Verification items for the finished model (mm, model axes). A direction names the side the tool comes from. Coordinates: 2 decimals unless noted, no trailing zeros. Write each loop counter-clockwise with the first axis right and the second up, starting at its lowest first coordinate (ties: lowest second). Pieces come first, ordered by that corner, then holes. Notation, with made-up numbers: (72.25, -7) - (97.25, -7) arc R25 cw to (97.25, 31) - close; hole circle Ø8 at (24.5, 18). An arc over 180 degrees is marked (long way). Answer as CSV lines item,"result". Start each with the question number.
```python
from build123d import *

# Parameters (mm, degrees)
SKETCH1_W           = 100
SKETCH1_H           = 100
SKETCH1_R           = 16.5
BOSS_EXTRUDE1_DEPTH = 10
SKETCH3_W           = 80
SKETCH3_H           = 80
SKETCH3_W_2         = 72
SKETCH3_H_2         = 72
BOSS_EXTRUDE2_DEPTH = 10


with BuildPart() as part:
    # Sketch1 → Boss-Extrude1 (new body)
    with BuildSketch(Plane(origin=(0, 0, 0), x_dir=(1, 0, 0), z_dir=(0, 1, 0))):
        Rectangle(SKETCH1_W, SKETCH1_H)
        with Locations(Location((0, 0, 0), (0, 0, 270))):
            Circle(SKETCH1_R, mode=Mode.SUBTRACT)
    extrude(amount=BOSS_EXTRUDE1_DEPTH)

    # Sketch3 → Boss-Extrude2 (add)
    with BuildSketch(Plane.XZ):
        Rectangle(SKETCH3_W, SKETCH3_H)
        Rectangle(SKETCH3_W_2, SKETCH3_H_2, mode=Mode.SUBTRACT)
    extrude(amount=BOSS_EXTRUDE2_DEPTH)


solid = part.part
```
1. Cross-section at B-B (x = 0). Record the cut outline in (y, z).
2. Cross-section at C-C (y = -7). Record the cut outline in (x, z), and give its area (3 significant figures).
3. Scan lines: line 1 along X through (y, z) = (4.75, 0); line 2 along Z through (x, y) = (4, -3.5). Record each from-to range of solid material in increasing order. Write a range as from..to.
4. Depth check by flat-ended pin: P1, Ø8, axis at y = -5.5, z = 12, coming from the -X side; P2, Ø1, axis at y = -6.5, z = -36, coming from the +X side; P3, Ø10, axis at x = 19.5, z = 12.5, coming from the -Y side. Enter the tip coordinate at first touch or a pass-through.
5. Access from +Z, -Z, +X, -X, +Y, -Y to the whole of each face (thin tool, end or side, straight path). Record for faces 4 (the face through (-1, -5, 40)), 5 (the face through (-12, 10, -12)), 6 (the face through (-3, -10, -38)), 7 (the face through (-1, -5, -40)), 8 (the face through (-17, 0, -1)).
6. Cross-section at D-D (z = -18). Record the cut outline in (x, y), and give its area (3 significant figures).
7. Draft check along X on faces 1 (the face through (40, -5, -1)), 2 (the face through (-1, -5, -36)), 3 (the face through (-40, -5, -1)). Enter one of: pulls with the +X half, pulls with the -X half, needs draft (parallel to the pull), parting line crosses it, or undercut.
8. Cross-section at A-A (z = 0). Record the cut outline in (x, y), and give its area (3 significant figures).
Completed:
1,outline,"(-10, -40) - (0, -40) - (0, -50) - (10, -50) - (10, -16.5) - (0, -16.5) - (0, -36) - (-10, -36) - close; (-10, 36) - (0, 36) - (0, 16.5) - (10, 16.5) - (10, 50) - (0, 50) - (0, 40) - (-10, 40) - close"
2,outline,"(-40, -40) - (40, -40) - (40, 40) - (-40, 40) - close; hole (-36, -36) - (36, -36) - (36, 36) - (-36, 36) - close"
2,area,"1,220 mm2"
3,line 1,"x = -50..-16.5, 16.5..50"
3,line 2,"z = -40..-36, 36..40"
4,P1,"stops at x = -40"
4,P2,"stops at x = 40"
4,P3,"stops at y = 0"
5,face 4,"+Z, +X, -X, -Y"
5,face 5,"+Z, -Z, +X, -X, +Y"
5,face 6,"+Z, -Z, +X, -X, -Y"
5,face 7,"-Z, +X, -X, -Y"
5,face 8,"-Y"
6,outline,"(-50, 0) - (-40, 0) - (-40, -10) - (-36, -10) - (-36, 0) - (36, 0) - (36, -10) - (40, -10) - (40, 0) - (50, 0) - (50, 10) - (-50, 10) - close"
6,area,"1,080 mm2"
7,face 1,"pulls with the +X half"
7,face 2,"undercut"
7,face 3,"pulls with the -X half"
8,outline,"(-50, 0) - (-40, 0) - (-40, -10) - (-36, -10) - (-36, 0) - (-16.5, 0) - (-16.5, 10) - (-50, 10) - close; (16.5, 0) - (36, 0) - (36, -10) - (40, -10) - (40, 0) - (50, 0) - (50, 10) - (16.5, 10) - close"
8,area,"750 mm2"
